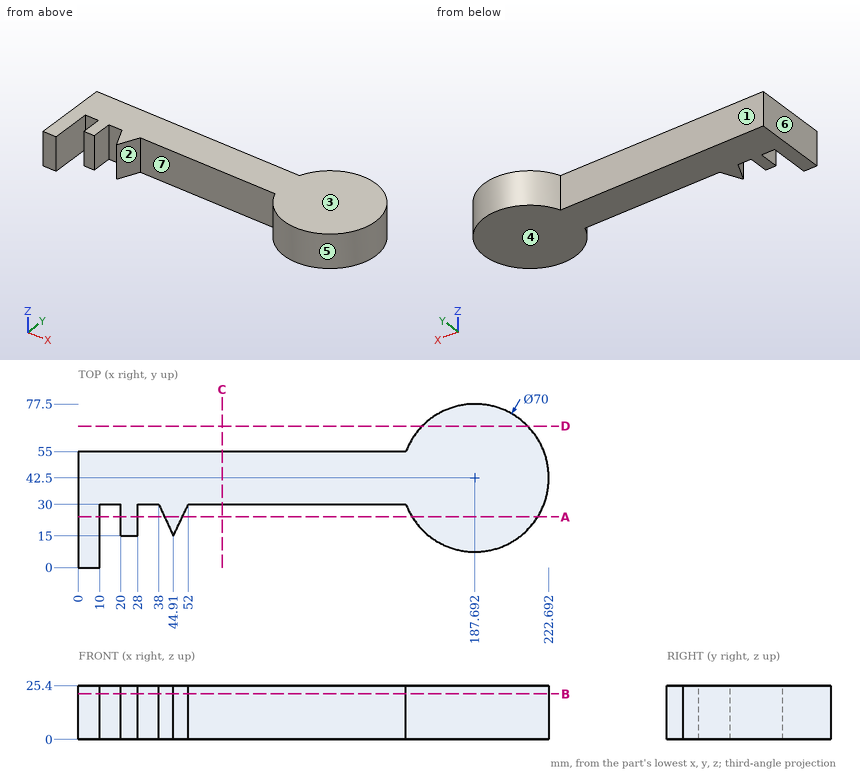
The drawing under review shows one solid part. Ordinate dimensions are in mm from its lowest x, y, z. A direction names the side the tool comes from. Coordinates: 2 decimals unless noted, no trailing zeros. Write each loop counter-clockwise with the first axis right and the second up, starting at its lowest first coordinate (ties: lowest second). Pieces come first, ordered by that corner, then holes. Notation, with made-up numbers: (-3.75, 76.25) -> (12.25, 76.25) arc R21 ccw to (12.25, 96.25) -> close; hole circle Ø11 at (86.25, 54). An arc over 180 degrees is marked (long way). One line per item, written item: value. Start each with the question number.
Q1. The part is to be moulded in two halves that separate along X. For the marked faces 4, 5, 6 and 7, say which applies: +X half, -X half, draft (parallel to the pull), parting line (faces both ways), or undercut.
Q2. Add section A-A, the plane y = 24. Give the boundary of the cut face in (x, z).
Q3. Add section C-C, the plane x = 68. Give the boundary of the cut face in (y, z), then the cut area to 3 significant figures.
Q4. Add section B-B, the plane z = 21.5. Give the boundary of the cut face in (x, y).
Q5. Clearance check with flat-ended pins moving along their axes: P1, Ø3, axis at x = 33.5, z = 10.5, coming from the -Y side; P2, Ø2, axis at y = 60.5, z = 22.5, coming from the +X side (1 decimal); P3, Ø2, axis at y = 27, z = 7, coming from the +X side. State where each tip first meets the part, or that it passes through.
Q6. To check wall thickness, follow probe 1 along X at (y, z) = (20, 9.5) (1 decimal); probe 2 along X at (y, z) = (25, 13.5) (1 decimal); probe 3 along Y at (x, z) = (68, 9.5). State the ranges of each line that lie inside material, in increasing order.
Q7. Add section D-D, the plane y = 67. Give the boundary of the cut face in (x, z), then the cut area to 3 significant figures.
Q8. For the marked faces 1, 2 and 3, list the 3-axis set-ups (+Z, -Z, +X, -X, +Y, -Y) from which the entire face can be reached by the end or side of a thin tool; tool diameter is ignored.
Response:
1. face 4: draft
1. face 5: undercut
1. face 6: -X half
1. face 7: undercut
2. outline: (0, 0) -> (10, 0) -> (10, 25.4) -> (0, 25.4) -> close; (20, 0) -> (28, 0) -> (28, 25.4) -> (20, 25.4) -> close; (40.76, 0) -> (49.16, 0) -> (49.16, 25.4) -> (40.76, 25.4) -> close; (157.98, 0) -> (217.4, 0) -> (217.4, 25.4) -> (157.98, 25.4) -> close
3. outline: (30, 0) -> (55, 0) -> (55, 25.4) -> (30, 25.4) -> close
3. area: 635 mm²
4. outline: (0, 0) -> (10, 0) -> (10, 30) -> (20, 30) -> (20, 15) -> (28, 15) -> (28, 30) -> (38, 30) -> (44.91, 15) -> (52, 30) -> (155, 30) arc R35 ccw (long way) to (155, 55) -> (0, 55) -> close
5. P1: y = 30
5. P2: x = 218.3
5. P3: x = 219.55
6. probe 1: 0 to 10, 20 to 28, 42.6 to 47.3, 160.9 to 214.5
6. probe 2: 0 to 10, 20 to 28, 40.3 to 49.6, 157.4 to 218
6. probe 3: 30 to 55
7. outline: (162.7, 0) -> (212.69, 0) -> (212.69, 25.4) -> (162.7, 25.4) -> close
7. area: 1,270 mm²
8. face 1: +Z, -Z, -X, +Y
8. face 2: +Z, -Z, -Y
8. face 3: +Z, +X, -X, +Y, -Y
